```python
from build123d import *

# Parameters (mm, degrees)
ESBO_O1_R                = 2
ESBO_O1_R_2              = 1.025
ESBO_O1_W                = 29.025
ESBO_O1_H                = 59.55
RESSALTO_EXTRUS_O2_DEPTH = 3
CHANFRO1_SIZE            = 0.325


with BuildPart() as part:
    # Esboço1 → Ressalto-extrusão2 (new body)
    with BuildSketch(Plane.XY):
        with BuildLine():
            Line((-20.103801855, 0.75392245), (-20.103801855, -138))
            Line((-20.103801855, -138), (-50.103801855, -138))
            Line((-50.103801855, -138), (-50.103801855, -188))
            Line((-50.103801855, -188), (50.096198145, -188))
            Line((50.096198145, -188), (50.096198145, -138))
            Line((50.096198145, -138), (20.096198145, -138))
            Line((20.096198145, -138), (20.096198145, -0.390922156))
            ThreePointArc((20.096198145, -0.390922156), (0.585154384, 20.862071726), (-20.103801855, 0.75392245))
        make_face()
        with Locations((45.096198145, -143)):
            Circle(ESBO_O1_R, mode=Mode.SUBTRACT)
        with Locations((45.096198145, -183)):
            Circle(ESBO_O1_R, mode=Mode.SUBTRACT)
        with Locations((-45.096198145, -183)):
            Circle(ESBO_O1_R, mode=Mode.SUBTRACT)
        with Locations((-45.096198145, -143)):
            Circle(ESBO_O1_R, mode=Mode.SUBTRACT)
        with Locations((14.516198145, -75.169414559)):
            Circle(ESBO_O1_R, mode=Mode.SUBTRACT)
        with Locations((14.516198145, -117.953999713)):
            Circle(ESBO_O1_R, mode=Mode.SUBTRACT)
        with Locations((-14.516198145, -117.953999713)):
            Circle(ESBO_O1_R, mode=Mode.SUBTRACT)
        with Locations((-14.516198145, -75.169414559)):
            Circle(ESBO_O1_R, mode=Mode.SUBTRACT)
        with Locations((17.325, -9.74607755)):
            Circle(ESBO_O1_R_2, mode=Mode.SUBTRACT)
        with Locations((-17.325, -9.74607755)):
            Circle(ESBO_O1_R_2, mode=Mode.SUBTRACT)
        with Locations((17.3125, -31.746073996)):
            Circle(ESBO_O1_R_2, mode=Mode.SUBTRACT)
        with Locations((17.3, -53.746070443)):
            Circle(ESBO_O1_R_2, mode=Mode.SUBTRACT)
        with Locations((-17.3, -53.746070443)):
            Circle(ESBO_O1_R_2, mode=Mode.SUBTRACT)
        with Locations((-17.3125, -31.746073996)):
            Circle(ESBO_O1_R_2, mode=Mode.SUBTRACT)
        with Locations((11, -61.546070443)):
            Circle(ESBO_O1_R_2, mode=Mode.SUBTRACT)
        with Locations((-11, -61.546070443)):
            Circle(ESBO_O1_R_2, mode=Mode.SUBTRACT)
        with Locations((0.0125, -29.02107755)):
            Rectangle(ESBO_O1_W, ESBO_O1_H, mode=Mode.SUBTRACT)
    extrude(amount=RESSALTO_EXTRUS_O2_DEPTH)

    # Chanfro1
    chanfro1_edges = [part.edges().sort_by_distance(p)[0] for p in [
        (16.2875, -31.746073996, 3),
        (16.275, -53.746070443, 3),
        (-18.325, -53.746070443, 3),
        (9.975, -61.546070443, 3),
        (-12.025, -61.546070443, 3),
        (-18.3375, -31.746073996, 3),
        (-18.35, -9.74607755, 3),
        (16.3, -9.74607755, 3),
    ]]
    chamfer(chanfro1_edges, length=CHANFRO1_SIZE)


solid = part.part
```
Input: part model. Units: mm. Frame: model coordinates. Give positions to 0.01 mm unless a question says otherwise; leave off trailing zeros. Order: outer loops, then holes, each group sorted by start corner. A loop starts at its lowest first (then second) coordinate and runs counter-clockwise, first axis right, second up. Notation, with made-up numbers: (-25, -15.5) - (-5, -15.5) arc R31 ccw to (-5, 14.5) - close; hole circle Ø3 at (47, -27.75). An arc over 180 degrees is marked (long way). Put each result on its own line as item: value.
Item 1: Ray query, L1, parallel to X at y = -32, z = 2.05 (3 decimals); L2, parallel to X at y = -183, z = 1.15; L3, parallel to X at y = -23.5, z = 1.35 (3 decimals). Return the intervals inside material, ascending. Write a range as from..to.
Found:
L1: x = -20.104..-18.306, -16.319..-14.5, 14.525..16.319, 18.306..20.096
L2: x = -50.1..-47.1, -43.1..43.1, 47.1..50.1
L3: x = -20.104..-14.5, 14.525..20.096
Item 2: Section query B-B, the plane x = 3. Return loops of the section in (y, z), then the cut area to 3 significant figures.
Found:
outline: (-188, 0) - (-58.8, 0) - (-58.8, 3) - (-188, 3) - close; (0.75, 0) - (20.65, 0) - (20.65, 3) - (0.75, 3) - close
area: 447 mm^2
Item 3: Contact query for flat-ended pins moving along their axis: pin 1 (0.9 mm diameter, centred on x = -35.5, z = 2, fed in from +Y); pin 2 (1.5 mm diameter, centred on x = 6, z = 1.5, fed in from +Y); pin 3 (1.5 mm diameter, centred on y = -24, z = 2.5, fed in from -X). Output: stop coordinate, or through.
Found:
pin 1: stops at y = -138
pin 2: stops at y = 20.18
pin 3: stops at x = -20.1
Item 4: Section query A-A, the plane y = -20. Return loops of the section in (x, z) (3 decimals), then the cut area to 3 significant figures.
Found:
outline: (-20.104, 0) - (-14.5, 0) - (-14.5, 3) - (-20.104, 3) - close; (14.525, 0) - (20.096, 0) - (20.096, 3) - (14.525, 3) - close
area: 33.5 mm^2
Item 5: Draft query along X for faces 1 (the cylindrical face through (-14.777, -73.186, 1.479)), 2 (the flat face through (-1, -129, 3)), 3 (the cylindrical face through (1.035, 20.844, 1.479)). Return one class per face: +X half, -X half, draft (parallel to the pull), parting line (faces both ways), or undercut.
Found:
face 1: undercut
face 2: draft
face 3: parting line
Item 6: Section query C-C, the plane y = -183. Return loops of the section in (x, z).
Found:
outline: (-50.1, 0) - (-47.1, 0) - (-47.1, 3) - (-50.1, 3) - close; (-43.1, 0) - (43.1, 0) - (43.1, 3) - (-43.1, 3) - close; (47.1, 0) - (50.1, 0) - (50.1, 3) - (47.1, 3) - close
Item 7: Section query D-D, the plane z = 1.15. Count the separate pieces of the cut face and the enclosed holes in it, then the cut area to 3 significant figures.
Found:
separate pieces: 1
enclosed holes: 17
area: 9,370 mm^2
